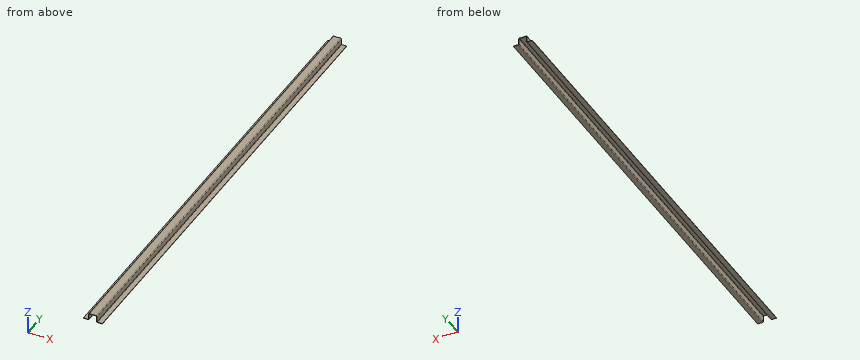
```python
from build123d import *

# Parameters (mm, degrees)
SKETCH1_W                      = 45
SKETCH1_H                      = 2508
BASE_FLANGE1_DEPTH             = 2
EDGE_FLANGE1_STRIP_W           = 13
EDGE_FLANGE1_STRIP_H           = 2
EDGE_FLANGE1_STRIP_CUT_DEPTH   = 2508
EDGE_FLANGE1_STRIP_2_W         = 13
EDGE_FLANGE1_STRIP_2_H         = 2
EDGE_FLANGE1_STRIP_CUT_2_DEPTH = 2508
EDGE_FLANGE1_DEPTH             = 2508
EDGE_FLANGE1_BEND_DEPTH        = 2508
EDGE_FLANGE2_STRIP_W           = 13
EDGE_FLANGE2_STRIP_H           = 2
EDGE_FLANGE2_STRIP_CUT_DEPTH   = 2508
EDGE_FLANGE2_STRIP_2_W         = 13
EDGE_FLANGE2_STRIP_2_H         = 2
EDGE_FLANGE2_STRIP_CUT_2_DEPTH = 2508
EDGE_FLANGE2_DEPTH             = 2508
EDGE_FLANGE2_BEND_DEPTH        = 2508


# Sheet-metal steps are written as plain solids
with BuildPart() as part:
    # Sketch1 → Base-Flange1 (new body)
    with BuildSketch(Plane.XY):
        Rectangle(SKETCH1_W, SKETCH1_H)
    extrude(amount=-BASE_FLANGE1_DEPTH)

    # Edge-Flange1 strip (across the edge) → Edge-Flange1 strip cut (cut)
    with BuildSketch(Plane(origin=(22.5, 1254, -2), x_dir=(-1, 0, 0), z_dir=(0, -1, 0))):
        with Locations((-2, -1)):
            Rectangle(EDGE_FLANGE1_STRIP_W, EDGE_FLANGE1_STRIP_H)
    extrude(amount=EDGE_FLANGE1_STRIP_CUT_DEPTH, mode=Mode.SUBTRACT)

    # Edge-Flange1 strip 2 (across the edge) → Edge-Flange1 strip cut 2 (cut)
    with BuildSketch(Plane(origin=(-22.5, -1254, -2), x_dir=(1, 0, 0), z_dir=(0, 1, 0))):
        with Locations((-2, -1)):
            Rectangle(EDGE_FLANGE1_STRIP_2_W, EDGE_FLANGE1_STRIP_2_H)
    extrude(amount=EDGE_FLANGE1_STRIP_CUT_2_DEPTH, mode=Mode.SUBTRACT)

    # Edge-Flange1 section (across the edge) → Edge-Flange1 (add)
    with BuildSketch(Plane(origin=(22.5, 1254, -2), x_dir=(-1, 0, 0), z_dir=(0, -1, 0))):
        with BuildLine():
            Line((0, 2.5), (0, 36))
            Line((0, 36), (2, 36))
            Line((2, 36), (2, 2.5))
            ThreePointArc((2, 2.5), (2.732233047, 0.732233047), (4.5, 0))
            Line((4.5, 0), (4.5, -2))
            ThreePointArc((4.5, -2), (1.318019485, -0.681980515), (0, 2.5))
        make_face()
    extrude(amount=EDGE_FLANGE1_DEPTH)

    # Edge-Flange1 section 2 (across the edge) → Edge-Flange1 bend (add)
    with BuildSketch(Plane(origin=(-22.5, -1254, -2), x_dir=(1, 0, 0), z_dir=(0, 1, 0))):
        with BuildLine():
            Line((0, 2.5), (0, 36))
            Line((0, 36), (2, 36))
            Line((2, 36), (2, 2.5))
            ThreePointArc((2, 2.5), (2.732233047, 0.732233047), (4.5, 0))
            Line((4.5, 0), (4.5, -2))
            ThreePointArc((4.5, -2), (1.318019485, -0.681980515), (0, 2.5))
        make_face()
    extrude(amount=EDGE_FLANGE1_BEND_DEPTH)

    # Edge-Flange2 strip (across the edge) → Edge-Flange2 strip cut (cut)
    with BuildSketch(Plane(origin=(-22.5, 1254, -38), x_dir=(0, 0, 1), z_dir=(0, -1, 0))):
        with Locations((-2, -1)):
            Rectangle(EDGE_FLANGE2_STRIP_W, EDGE_FLANGE2_STRIP_H)
    extrude(amount=EDGE_FLANGE2_STRIP_CUT_DEPTH, mode=Mode.SUBTRACT)

    # Edge-Flange2 strip 2 (across the edge) → Edge-Flange2 strip cut 2 (cut)
    with BuildSketch(Plane(origin=(22.5, -1254, -38), x_dir=(0, 0, 1), z_dir=(0, 1, 0))):
        with Locations((-2, -1)):
            Rectangle(EDGE_FLANGE2_STRIP_2_W, EDGE_FLANGE2_STRIP_2_H)
    extrude(amount=EDGE_FLANGE2_STRIP_CUT_2_DEPTH, mode=Mode.SUBTRACT)

    # Edge-Flange2 section (across the edge) → Edge-Flange2 (add)
    with BuildSketch(Plane(origin=(-22.5, 1254, -38), x_dir=(0, 0, 1), z_dir=(0, -1, 0))):
        with BuildLine():
            Line((0, 2.5), (0, 28))
            Line((0, 28), (2, 28))
            Line((2, 28), (2, 2.5))
            ThreePointArc((2, 2.5), (2.732233047, 0.732233047), (4.5, 0))
            Line((4.5, 0), (4.5, -2))
            ThreePointArc((4.5, -2), (1.318019485, -0.681980515), (0, 2.5))
        make_face()
    extrude(amount=EDGE_FLANGE2_DEPTH)

    # Edge-Flange2 section 2 (across the edge) → Edge-Flange2 bend (add)
    with BuildSketch(Plane(origin=(22.5, -1254, -38), x_dir=(0, 0, 1), z_dir=(0, 1, 0))):
        with BuildLine():
            Line((0, 2.5), (0, 28))
            Line((0, 28), (2, 28))
            Line((2, 28), (2, 2.5))
            ThreePointArc((2, 2.5), (2.732233047, 0.732233047), (4.5, 0))
            Line((4.5, 0), (4.5, -2))
            ThreePointArc((4.5, -2), (1.318019485, -0.681980515), (0, 2.5))
        make_face()
    extrude(amount=EDGE_FLANGE2_BEND_DEPTH)


solid = part.part
```
Design review of the part built by this model. Coordinates are the model's own, in mm. Round coordinates to 2 decimals unless told otherwise and drop trailing zeros. Write each loop counter-clockwise with the first axis right and the second up, starting at its lowest first coordinate (ties: lowest second). Pieces come first, ordered by that corner, then holes.
Item 1: We need section A-A on z = -21. Write out the cut boundary in (x, y), and give its area (3 significant figures).
Item 2: We need section B-B on y = 198. Write out the cut boundary in (x, z).
Item 3: Clearance check with flat-ended pins moving along their axes: pin 1 Ø1 at (x, y) = (-13, 546.5) entering from -Z; pin 2 Ø14.5 at (y, z) = (447.5, -12) entering from +X; pin 3 Ø8.5 at (y, z) = (-181, -25) entering from -X; pin 4 Ø3 at (x, y) = (-8.5, 42) entering from +Z. State where each tip first meets the part, or that it passes through.
Item 4: We need section C-C on x = 2. Write out the cut boundary in (y, z), and give its area (3 significant figures).
Item 5: For probe 1 along X at (y, z) = (858, -31); probe 2 along Z at (x, y) = (-4, -469); probe 3 along Z at (x, y) = (39.5, 741.5), list the stretches that pass through material, from the lowest coordinate up.
Returned:
1. outline: (-22.5, -1254) - (-20.5, -1254) - (-20.5, 1254) - (-22.5, 1254) - close; (20.5, -1254) - (22.5, -1254) - (22.5, 1254) - (20.5, 1254) - close
1. area: 10,000 mm2
2. outline: (-50.5, -38) - (-25, -38) arc R4.5 ccw to (-20.5, -33.5) - (-20.5, -4.5) arc R2.5 cw to (-18, -2) - (18, -2) arc R2.5 cw to (20.5, -4.5) - (20.5, -33.5) arc R4.5 ccw to (25, -38) - (50.5, -38) - (50.5, -36) - (25, -36) arc R2.5 cw to (22.5, -33.5) - (22.5, -4.5) arc R4.5 ccw to (18, 0) - (-18, 0) arc R4.5 ccw to (-22.5, -4.5) - (-22.5, -33.5) arc R2.5 cw to (-25, -36) - (-50.5, -36) - close
3. pin 1: stops at z = -2
3. pin 2: stops at x = 22.5
3. pin 3: stops at x = -22.5
3. pin 4: stops at z = 0
4. outline: (-1254, -2) - (1254, -2) - (1254, 0) - (-1254, 0) - close
4. area: 5,020 mm2
5. probe 1: x = -22.5 to -20.5, 20.5 to 22.5
5. probe 2: z = -2 to 0
5. probe 3: z = -38 to -36
